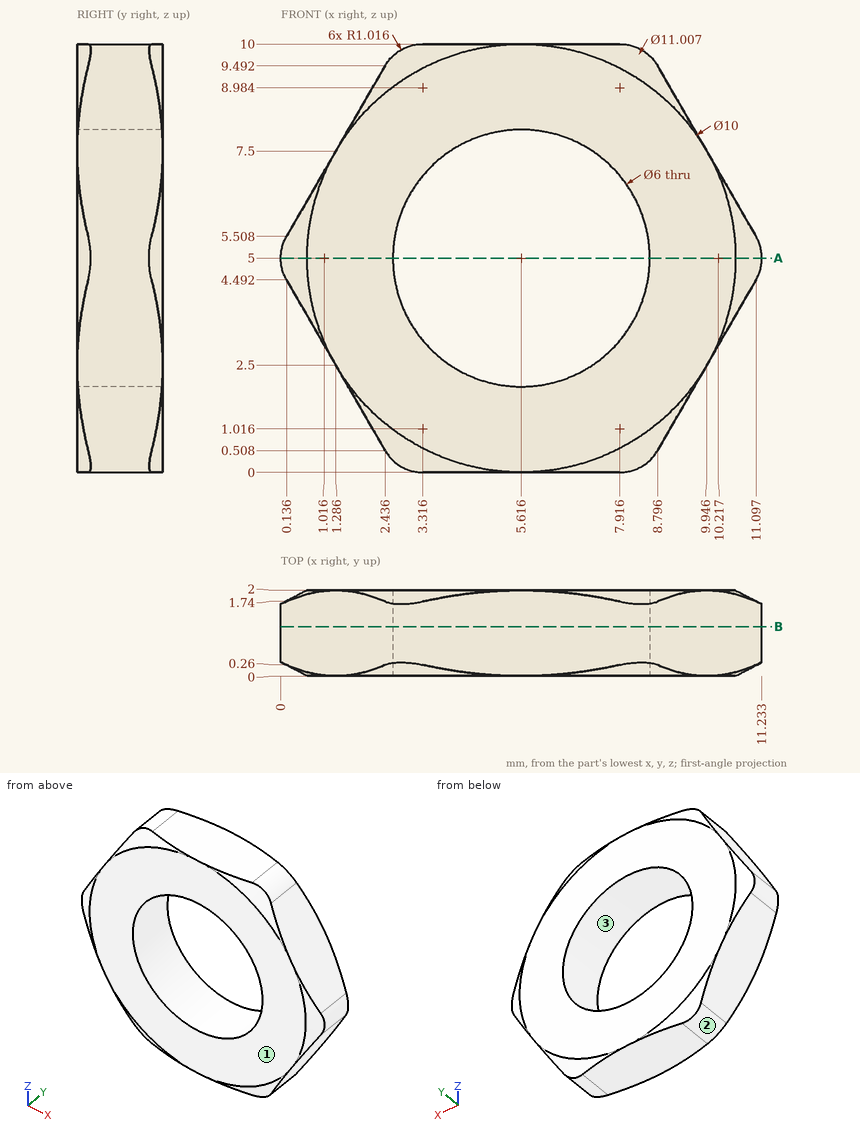
Could you check a few things on this drawing? It's one solid part, dimensions in mm from its lowest x, y, z. Coordinates: 2 decimals unless noted, no trailing zeros. Order: outer loops, then holes, each group sorted by start corner. A loop starts at its lowest first (then second) coordinate and runs counter-clockwise, first axis right, second up. Notation, with made-up numbers: (49.25, -37.75) - (55.25, -37.75) arc R15 ccw to (55.25, -9.75) - close; hole circle Ø9 at (-38.75, -26.75). An arc over 180 degrees is marked (long way). One line per question, with ' | ' between items. Start each with the question number.
1. I'm going to push a flat-ended pin straight in: pin 1 Ø3.5 at (x, z) = (5.62, 5) entering from -Y. Where does the tip first touch, or does it pass through?
2. If we section it at B-B (y = 1.15): Write out the boundary of the cut face in (x, z).
3. If we section it at A-A (z = 5): Write out the boundary of the cut face in (x, y).
4. Please list where these lines run through material, in increasing order: line 1 along Z through (x, y) = (8, 1.6) (1 decimal); line 2 along X through (y, z) = (0.75, 6.5) (1 decimal); line 3 along Z through (x, y) = (4.25, 1.45). Write a range as [from, to].
5. If we mould it in two halves opening along X, with no side actions, what happens to the marked faces 1, 2 and 3? For each: released by +X, released by -X, zero draft, split by the parting line, or undercut.
Model answer:
1) pin 1: passes through
2) outline: (0.14, 4.49) - (2.44, 0.51) arc R1.02 ccw to (3.32, 0) - (7.92, 0) arc R1.02 ccw to (8.8, 0.51) - (11.1, 4.49) arc R1.02 ccw to (11.1, 5.51) - (8.8, 9.49) arc R1.02 ccw to (7.92, 10) - (3.32, 10) arc R1.02 ccw to (2.44, 9.49) - (0.14, 5.51) arc R1.02 ccw to start; hole circle Ø6 at (5.62, 5)
3) outline: (0, 0.32) - (0.62, 0) - (2.62, 0) - (2.62, 2) - (0.62, 2) - (0, 1.68) - close; (8.62, 0) - (10.62, 0) - (11.23, 0.32) - (11.23, 1.68) - (10.62, 2) - (8.62, 2) - close
4) line 1: z = [0, 3.2], [6.8, 10] | line 2: x = [0.7, 3], [8.2, 10.5] | line 3: z = [0, 2.33], [7.67, 10]
5) face 1: zero draft | face 2: released by -X | face 3: undercut
